The model under review builds one solid part; all positions refer to its coordinate system, in mm. Face numbers are marked on the shaded views. A direction names the side the tool comes from. Round coordinates to 2 decimals unless told otherwise and drop trailing zeros. Loops run counter-clockwise (first coordinate to the right, second up) from the corner with the lowest first, then second, coordinate; pieces in that order, holes last. Notation, with made-up numbers: (4, -2) -> (21, -2) arc R23 ccw to (21, 6) -> close; hole circle Ø8 at (11.25, 62). An arc over 180 degrees is marked (long way). Use a Markdown table: item, result. Add a question column.
1) For the marked faces 1, 2 and 3, list the 3-axis set-ups (+Z, -Z, +X, -X, +Y, -Y) from which the entire face can be reached by the end or side of a thin tool; tool diameter is ignored.
2) Consider section A-A on y = 4.5. Give the boundary of the cut face in (x, z).
3) Consider section C-C on x = -13. Give the boundary of the cut face in (y, z), plus the area to 3 significant figures.
4) Consider section D-D on y = 35.5. Give the boundary of the cut face in (x, z), plus the area to 3 significant figures.
5) Consider section B-B on z = 6.5. Give the boundary of the cut face in (x, y), plus the area to 3 significant figures.
6) Mouldability with a two-part tool opening along X and no side actions: class the marked faces 4, 5 and 6 as released by +X, released by -X, zero draft, split by the parting line, or undercut.
7) Insertion check: pin 1 (2.5 mm diameter, centred on y = 39, z = 37, fed in from -X); pin 2 (1.5 mm diameter, centred on x = -18.5, y = 16, fed in from -Z); pin 3 (5 mm diameter, centred on x = 23.5, z = 21.5, fed in from -Y); pin 4 (2 mm diameter, centred on x = 34, z = 40.5, fed in from -Y). Each pin has a flat end and moves straight along its axis. Give the tip position at first contact, or say it passes through.
8) Wall thickness on probe 1 along X at (y, z) = (33.5, 21.5); probe 2 along X at (y, z) = (26, 26); probe 3 along Y at (x, z) = (23, 45.5): over which ranges is each line inside the solid? List them lowest first.
from build123d import *

# Parameters (mm, degrees)
F0_R     = 11
F1_DEPTH = 10
F3_D     = 3
F0_W     = 10
F0_H     = 9.75
F0_W_2   = 20
F4_DEPTH = 50
F5_R     = 1.5
F6_DEPTH = 3
F7_DEPTH = 20


with BuildPart() as f1:
    # F0 (on Top) → F1 (new body)
    with BuildSketch(Plane.XY):
        Polygon((18.0623630062, 45), (-31.9376369938, 45), (-31.9376369938, -5), (18.0623630062, -5), (18.0623630062, 0), (18.0623630062, 20.5), (18.0623630062, 30.25), (18.0623630062, 40), align=None)
        with Locations((-6.9376369938, 20)):
            Circle(F0_R, mode=Mode.SUBTRACT)
    extrude(amount=F1_DEPTH)

    # F3 (through all)
    with Locations(Plane(origin=(0, 0, 0), x_dir=(1, 0, 0), z_dir=(0, 0, -1))):
        with Locations((8.5623630062, -4.5), (-22.4376369938, -4.5), (-22.4376369938, -35.5), (8.5623630062, -35.5)):
            Hole(F3_D / 2)

    # F0 (on Top) → F4 (join)
    with BuildSketch(Plane.XY):
        with Locations((23.0623630062, 25.375)):
            Rectangle(F0_W, F0_H)
        with Locations((23.0623630062, 35.125)):
            Rectangle(F0_W, F0_H)
        with Locations((38.0623630062, 35.125)):
            Rectangle(F0_W_2, F0_H)
        with Locations((53.0623630062, 35.125)):
            Rectangle(F0_W, F0_H)
        with Locations((53.0623630062, 25.375)):
            Rectangle(F0_W, F0_H)
    extrude(amount=F4_DEPTH)

    # F5 (on face) → F6 (cut)
    with BuildSketch(Plane(origin=(0, 40, 0), x_dir=(-1, 0, 0), z_dir=(0, 1, 0))):
        Polygon((-20.0623630062, 25.1961524227), (-23.0623630062, 26.9282032303), (-26.0623630062, 25.1961524227), (-26.0623630062, 21.7320508076), (-23.0623630062, 20), (-20.0623630062, 21.7320508076), align=None)
        with Locations((-23.0623630062, 23.4641016151)):
            Circle(F5_R, mode=Mode.SUBTRACT)
        Polygon((-20.0623630062, 38.2679491924), (-23.0623630062, 40), (-26.0623630062, 38.2679491924), (-26.0623630062, 34.8038475773), (-23.0623630062, 33.0717967697), (-20.0623630062, 34.8038475773), align=None)
        with Locations((-23.0623630062, 36.5358983849)):
            Circle(F5_R, mode=Mode.SUBTRACT)
        Polygon((-56.0623630062, 34.8038475773), (-53.0623630062, 33.0717967697), (-50.0623630062, 34.8038475773), (-50.0623630062, 38.2679491924), (-53.0623630062, 40), (-56.0623630062, 38.2679491924), align=None)
        with Locations((-53.0623630062, 36.5358983849)):
            Circle(F5_R, mode=Mode.SUBTRACT)
        Polygon((-56.0623630062, 21.7320508076), (-53.0623630062, 20), (-50.0623630062, 21.7320508076), (-50.0623630062, 25.1961524227), (-53.0623630062, 26.9282032303), (-56.0623630062, 25.1961524227), align=None)
        with Locations((-53.0623630062, 23.4641016151)):
            Circle(F5_R, mode=Mode.SUBTRACT)
    extrude(amount=-F6_DEPTH, mode=Mode.SUBTRACT)

    # F7 (cut): faces of the model
    f7_faces = [f1.faces().sort_by_distance(p)[0] for p in [
        (23.0623630062, 40, 23.4641016151),
        (23.0623630062, 40, 36.5358983849),
        (53.0623630062, 40, 36.5358983849),
        (53.0623630062, 40, 23.4641016151),
    ]]
    extrude(f7_faces, amount=-F7_DEPTH, mode=Mode.SUBTRACT)


solid = f1.part
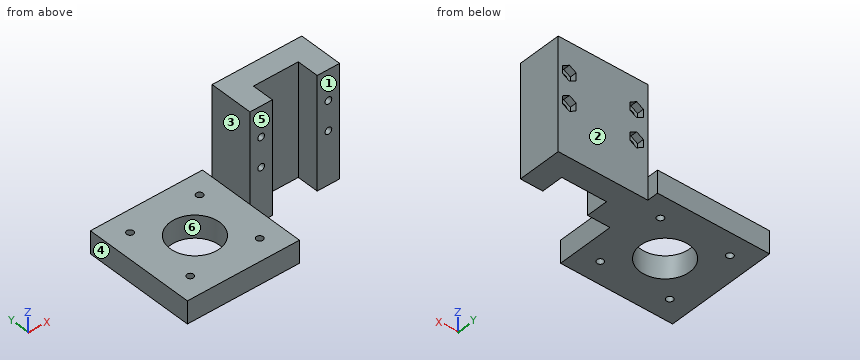
Result set:
| question | item | result |
|---|---|---|
| 1 | face 1 | +Z, -Z, +X, -Y |
| 1 | face 2 | +Z, -Z, +X, +Y |
| 1 | face 3 | +Z, -X, +Y, -Y |
| 2 | outline | (-31.94, 0) -> (-23.94, 0) -> (-23.94, 10) -> (-31.94, 10) -> close; (-20.94, 0) -> (7.06, 0) -> (7.06, 10) -> (-20.94, 10) -> close; (10.06, 0) -> (18.06, 0) -> (18.06, 10) -> (10.06, 10) -> close |
| 3 | outline | (-5, 0) -> (10.82, 0) -> (10.82, 10) -> (-5, 10) -> close; (29.18, 0) -> (45, 0) -> (45, 10) -> (29.18, 10) -> close |
| 3 | area | 316 mm2 |
| 4 | outline | (-31.94, 0) -> (-23.94, 0) -> (-23.94, 10) -> (-31.94, 10) -> close; (-20.94, 0) -> (7.06, 0) -> (7.06, 10) -> (-20.94, 10) -> close; (10.06, 0) -> (58.06, 0) -> (58.06, 50) -> (18.06, 50) -> (18.06, 10) -> (10.06, 10) -> close; hole circle Ø3 at (23.06, 23.46); hole circle Ø3 at (23.06, 36.54); hole circle Ø3 at (53.06, 23.46); hole circle Ø3 at (53.06, 36.54) |
| 4 | area | 2,410 mm2 |
| 5 | outline | (-31.94, -5) -> (18.06, -5) -> (18.06, 20.5) -> (28.06, 20.5) -> (28.06, 30.25) -> (48.06, 30.25) -> (48.06, 20.5) -> (58.06, 20.5) -> (58.06, 40) -> (18.06, 40) -> (18.06, 45) -> (-31.94, 45) -> close; hole circle Ø3 at (-22.44, 4.5); hole circle Ø3 at (-22.44, 35.5); hole circle Ø22 at (-6.94, 20); hole circle Ø3 at (8.56, 4.5); hole circle Ø3 at (8.56, 35.5) |
| 5 | area | 2,680 mm2 |
| 6 | face 4 | released by -X |
| 6 | face 5 | zero draft |
| 6 | face 6 | undercut |
| 7 | pin 1 | x = 18.06 |
| 7 | pin 2 | z = 0 |
| 7 | pin 3 | y = 20.5 |
| 7 | pin 4 | y = 30.25 |
| 8 | probe 1 | 18.06 to 58.06 |
| 8 | probe 2 | 18.06 to 28.06, 48.06 to 58.06 |
| 8 | probe 3 | 20.5 to 40 |
